Autodesk Inventor part; units mm, degrees
ref_plane "Work Plane1" through (4, 0, 0) normal (1, 0, 0) x (0, 1, 0)
ref_plane "XZ Plane" through (0, 0, 0) normal (0, 1, 0) x (-1, 0, 0)
ref_plane "XY Plane" through (0, 0, 0) normal (0, 0, 1) x (1, 0, 0)
sketch "Sketch1" plane through (0, 0, 0) normal (0, 0, 1) x (1, 0, 0)
  line L0 (0, 0) -> (0, 16.1) construction
  line L1 (0, 0) -> (4.1, 0) construction
  line L2 (4.1, 0) -> (4.1, 16.1)
  line L3 (4.1, 16.1) -> (0, 16.1) construction
  line L4 (4.1, 16.1) -> (17.5, 16.1) construction
  line L5 (17.5, 16.1) -> (17.5, 15.6)
  line L6 (17.5, 15.6) -> (16, 15.1)
  line L7 (16, 15.1) -> (16, 11.5)
  line L8 (16, 11.5) -> (17.5, 11)
  line L9 (17.5, 11) -> (17.5, 10)
  line L10 (17.5, 10) -> (9, 6)
  line L11 (9, 6) -> (9, 0)
  line L12 (9, 0) -> (4.1, 0)
  line L13 (9, 0) -> (5.1, -1) construction
  line L14 (5.1, -1) -> (4.1, -1) construction
  line L15 (4.1, -1) -> (4.1, 0) construction
  line L16 (4.1, 16.1) -> (4.1, 16.6)
  line L17 (4.1, 16.6) -> (5.1, 16.6) construction
  line L18 (5.1, 16.6) -> (17.5, 16.1)
  line L19 (5.1, 16.6) -> (5.1, 17.6)
  line L20 (5.1, 17.6) -> (4.1, 17.6)
  line L21 (4.1, 17.6) -> (4.1, 16.6)
  dimension "d0" = 4.1
  dimension "d1" = 3.6
  dimension "d2" = 0.5
  dimension "d3" = 1
  dimension "d4" = 0.5
  dimension "d5" = 1.5
  dimension "d6" = 9
  dimension "d7" = 16
  dimension "d8" = 4
  dimension "d9" = 6
  dimension "d11" = 1
  dimension "d12" = 1
  dimension "d13" = 1
  dimension "d14" = 0.5
  dimension "d15" = 1
revolve "Revolution1" add sketch "Sketch1" angle 360 about axis through (0, 0, 0) along (0, 1, 0)
ref_plane "Work Plane1" through (4, 0, 0) normal (1, 0, 0) x (0, 1, 0)
sketch "Sketch2" plane through (4, 0, 0) normal (1, 0, 0) x (0, 1, 0)
  line L0 (0, 0) -> (2.85, 0) construction
  line L1 (0, 2.85) -> (5.7, 2.85)
  line L2 (5.7, 2.85) -> (5.7, -2.85)
  line L3 (5.7, -2.85) -> (0, -2.85)
  line L4 (0, -2.85) -> (0, 2.85)
  line L5 (0, 2.85) -> (5.7, -2.85) construction
  line L6 (5.7, 2.85) -> (0, -2.85) construction
  line L7 (0, 4.1) -> (0, -4.1)
  dimension "d17" = 5.7
  dimension "d18" = 5.7
extrude "Extrusion1" cut sketch "Sketch2" along normal blind 2.5 and the other way blind 3
sketch "Sketch3" plane through (4, 0, 0) normal (1, 0, 0) x (0, 1, 0)
  line L0 (5.7, -2.85) -> (0, 2.85) construction
  circle A0 centre (2.85, 0) radius 1.7
  point P0 (0, 0)
  dimension "d23" = 3.4
extrude "Extrusion2" cut sketch "Sketch3" along normal through all
sketch "Sketch4" plane through (0, 0, 0) normal (0, -1, 0) x (1, 0, 0)
  circle A0 centre (0, 0) radius 26.9979
extrude "SetScrewDelete" cut sketch "Sketch4" against normal blind 10.5
chamfer "Chamfer1" distance 0.3 angle 45 1 edges at (-17.5, 10.5, 0)
properties part number "DrivenPulley"
Design review of the part built by this model. Coordinates are the model's own, in mm. Coordinates: 2 decimals unless noted, no trailing zeros. Loops run counter-clockwise (first coordinate to the right, second up) from the corner with the lowest first, then second, coordinate; pieces in that order, holes last. Notation, with made-up numbers: M -22.5,21 L -4.5,21 A32 ccw -4.5,47 Z; hole C 31.5,9.5 d8. An arc over 180 degrees is marked long. Answer as CSV lines item,"result".
Item 1: Add section A-A on x = 0. State the section outline as (y, z) points, plus the area to 3 significant figures.
Answer list:
outline,"M 10.5,-17.2 L 10.8,-17.5 L 11,-17.5 L 11.5,-16 L 15.1,-16 L 15.6,-17.5 L 16.1,-17.5 L 16.6,-5.1 L 17.6,-5.1 L 17.6,-4.1 L 10.5,-4.1 Z; M 10.5,4.1 L 17.6,4.1 L 17.6,5.1 L 16.6,5.1 L 16.1,17.5 L 15.6,17.5 L 15.1,16 L 11.5,16 L 11,17.5 L 10.8,17.5 L 10.5,17.2 Z"
area,"147 mm²"
Item 2: The part is to be moulded in two halves that separate along Y. For faces 1 (the face through (-3.47, 13.27, -15.62)), 2 (the face through (-1.27, 16.57, -5.74)), 3 (the face through (2.4, 17.1, 4.5)), say which applies: pulls with the +Y half, pulls with the -Y half, needs draft (parallel to the pull), parting line crosses it, or undercut.
Answer list:
face 1,"undercut"
face 2,"pulls with the +Y half"
face 3,"needs draft"
Item 3: For probe 1 along Z at (x, y) = (0, 13.75); probe 2 along X at (y, z) = (16, 0), list the stretches that pass through material, from the lowest coordinate up.
Answer list:
probe 1,"-16 to -4.1, 4.1 to 16"
probe 2,"-17.5 to -4.1, 4.1 to 17.5"
Item 4: Add section C-C on y = 12.25. State the section outline as (x, z) points, plus the area to 3 significant figures.
Answer list:
outline,"C 0,0 d32; hole C 0,0 d8.2"
area,"751 mm²"
Item 5: Add section B-B on z = 0. State the section outline as (x, y) points.
Answer list:
outline,"M -17.5,10.8 L -17.2,10.5 L -4.1,10.5 L -4.1,17.6 L -5.1,17.6 L -5.1,16.6 L -17.5,16.1 L -17.5,15.6 L -16,15.1 L -16,11.5 L -17.5,11 Z; M 4.1,10.5 L 17.2,10.5 L 17.5,10.8 L 17.5,11 L 16,11.5 L 16,15.1 L 17.5,15.6 L 17.5,16.1 L 5.1,16.6 L 5.1,17.6 L 4.1,17.6 Z"
Item 6: For P1, Ø1, axis at x = 1.5, y = 13, coming from the -Z side; P2, Ø4, axis at x = 7.5, z = 7.5, coming from the +Y side; P3, Ø4, axis at y = 14, z = -0.5, coming from the +X side; P4, Ø1.5, axis at y = 16.5, z = -5.5, coming from the +X side, all flat-tipped, find the tip position at first contact; note any pin that passes through.
Answer list:
P1,"z = -15.97"
P2,"y = 16.46"
P3,"x = 17.5"
P4,"x = 16.81"
